Model file for the job. Use its own axes, mm. A direction names the side the tool comes from. Coordinates: 2 decimals unless noted, no trailing zeros. Write each loop counter-clockwise with the first axis right and the second up, starting at its lowest first coordinate (ties: lowest second). Pieces come first, ordered by that corner, then holes. Notation, with made-up numbers: (-26.75, 43) -> (24.25, 43) arc R14 cw to (24.25, 54) -> close; hole circle Ø10 at (13.5, -19.75). An arc over 180 degrees is marked (long way). Answer as a JSON object with one key per item and string values. Group by question number.
from build123d import *

# Parameters (mm, degrees)
EXTRUDE_2_DEPTH             = 20
HOLE_WIZARD_M41_D           = 4.5
HOLE_WIZARD_M41_DEPTH       = 6
HOLE_WIZARD_M41_CBORE_D     = 8
HOLE_WIZARD_M41_CBORE_DEPTH = 4
M4X0_71_D                   = 3.3
FILLET_1_R                  = 2
FILLET_2_R                  = 4
M4X0_72_D                   = 3.3
FILLET_3_R                  = 3


with BuildPart() as part:
    # Эскиз1 → Бобышка-Вытянуть2 (new body)
    with BuildSketch(Plane.XY):
        with BuildLine():
            Line((-6.608514495, 10.45), (6.608514495, 10.45))
            ThreePointArc((6.608514495, 10.45), (14.066074726, 13.916265053), (22.186198751, 12.614810542))
            Line((22.186198751, 12.614810542), (34.177275866, 33.383965344))
            Line((34.177275866, 33.383965344), (47.167656923, 25.883965344))
            Line((47.167656923, 25.883965344), (28.167656923, -7.025))
            ThreePointArc((28.167656923, -7.025), (23.025, -12.167656923), (16, -14.05))
            Line((16, -14.05), (-16, -14.05))
            ThreePointArc((-16, -14.05), (-23.025, -12.167656923), (-28.167656923, -7.025))
            Line((-28.167656923, -7.025), (-47.167656923, 25.883965344))
            Line((-47.167656923, 25.883965344), (-34.177275866, 33.383965344))
            Line((-34.177275866, 33.383965344), (-22.186198751, 12.614810542))
            ThreePointArc((-22.186198751, 12.614810542), (-14.066074726, 13.916265053), (-6.608514495, 10.45))
        make_face()
        with BuildLine():
            Line((-5.885653753, 4.45), (5.885653753, 4.45))
            ThreePointArc((5.885653753, 4.45), (27.047875471, -0.216673901), (5.71894947, -4.05))
            Line((5.71894947, -4.05), (-5.71894947, -4.05))
            ThreePointArc((-5.71894947, -4.05), (-27.047875471, -0.216673901), (-5.885653753, 4.45))
        make_face(mode=Mode.SUBTRACT)
    extrude(amount=EXTRUDE_2_DEPTH)

    # Цековка для винта с внутренним шестигранником M41
    with Locations(Plane(origin=(0, 10.45, 0), x_dir=(1, 0, 0), z_dir=(0, 1, 0))):
        with Locations((0, -10)):
            CounterBoreHole(HOLE_WIZARD_M41_D / 2, HOLE_WIZARD_M41_CBORE_D / 2, HOLE_WIZARD_M41_CBORE_DEPTH, depth=HOLE_WIZARD_M41_DEPTH)

    # Отверстие обработанное метчиком M4x0.71 (through all)
    with Locations(Plane(origin=(0, -4.05, 0), x_dir=(1, 0, 0), z_dir=(0, 1, 0))):
        with Locations((0, -10)):
            Hole(M4X0_71_D / 2)

    # Скругление1
    fillet_1_edges = [part.edges().sort_by_distance(p)[0] for p in [
        (-5.885653753, 4.45, 10),
        (-5.71894947, -4.05, 10),
        (5.71894947, -4.05, 10),
        (5.885653753, 4.45, 10),
    ]]
    fillet(fillet_1_edges, radius=FILLET_1_R)

    # Скругление2
    fillet_2_edges = [part.edges().sort_by_distance(p)[0] for p in [
        (-6.608514495, 10.45, 10),
        (6.608514495, 10.45, 10),
        (22.186198751, 12.614810542, 10),
        (-22.186198751, 12.614810542, 10),
    ]]
    fillet(fillet_2_edges, radius=FILLET_2_R)

    # Отверстие обработанное метчиком M4x0.72 (through all)
    with Locations(Plane(origin=(24.167656923, -13.95320323, 0), x_dir=(0, 0, -1), z_dir=(0.866025404, -0.5, 0))):
        with Locations((-10, 26), (-16, 38)):
            m4x0_72 = Hole(M4X0_72_D / 2)

    # Зеркальное отражение1: Отверстие обработанное метчиком M4x0.72 across plane
    add(m4x0_72.mirror(Plane(origin=(0, 0, 0), x_dir=(0, 0, 1), z_dir=(1, 0, 0))), mode=Mode.SUBTRACT)

    # Скругление3
    fillet_3_edges = [part.edges().sort_by_distance(p)[0] for p in [
        (34.177275866, 33.383965344, 10),
        (47.167656923, 25.883965344, 10),
        (-47.167656923, 25.883965344, 10),
        (-34.177275866, 33.383965344, 10),
    ]]
    fillet(fillet_3_edges, radius=FILLET_3_R)


solid = part.part
(1) Wall check: probe 1 along Z at (x, y) = (0, -8); probe 2 along Z at (x, y) = (0, 9.1); probe 3 along X at (y, z) = (-4.5, 5). Give the ranges that are in metal, low to high.
(2) Pull direction Z, two halves, no side cores. Call faces 1 (the face through (-3, 9, 20)), 2 (the face through (-36.829, 23.187, 17.574)), 3 (the face through (37.04, 8.34, 7.64)): released by +Z, released by -Z, zero draft, split by the parting line, or undercut.
(3) Cut at B-B on y = 0.5. List the corners of the cut face in (x, z).
(4) Cut at C-C on z = 16.25. Give the number of separate pieces and of enclosed holes in the cut face, plus the area to 3 significant figures.
(5) Pin check, flat tips, straight feed: pin 1 (8 mm diameter, centred on x = 9, z = 9.5, fed in from +Y); pin 2 (3 mm diameter, centred on y = 11.5, z = 17.5, fed in from +X); pin 3 (2 mm diameter, centred on x = 1, z = 5, fed in from +Y); pin 4 (3 mm diameter, centred on x = 0, z = 10, fed in from -Y). Stop position of each tip, or through.
(6) Cut at A-A on x = 0. List the corners of the cut face in (y, z), plus the area to 3 significant figures.
(7) 3-axis set-ups, long thin cutter, end or side, ignore diameter. For faces 4 (the face through (28.205, 23.04, 9.86)), 5 (the face through (-0.1, 4.45, 7.6)), 6 (the face through (0.29, 5.44, 7.77)): which of +Z, -Z, +X, -X, +Y, -Y reach the whole face in a straight line?
Results found:
{
 "1": {"probe 1": "z = 0 to 8.35, 11.65 to 20", "probe 2": "z = 0 to 6, 14 to 20", "probe 3": "x = -29.63 to -26.09, -5.7 to 5.7, 26.09 to 29.63"},
 "2": {"face 1": "released by +Z", "face 2": "undercut", "face 3": "zero draft"},
 "3": {"outline": "(-32.51, 0) -> (-27.04, 0) -> (-27.04, 20) -> (-32.51, 20) -> close; (27.04, 0) -> (32.51, 0) -> (32.51, 20) -> (27.04, 20) -> close"},
 "4": {"separate pieces": "3", "enclosed holes": "1", "area": "1,300 mm²"},
 "5": {"pin 1": "stops at y = 13.73", "pin 2": "stops at x = 39.73", "pin 3": "stops at y = 10.45", "pin 4": "passes through"},
 "6": {"outline": "(-14.05, 0) -> (-4.05, 0) -> (-4.05, 8.35) -> (-14.05, 8.35) -> close; (-14.05, 11.65) -> (-4.05, 11.65) -> (-4.05, 20) -> (-14.05, 20) -> close; (4.45, 0) -> (10.45, 0) -> (10.45, 6) -> (6.45, 6) -> (6.45, 7.75) -> (4.45, 7.75) -> close; (4.45, 12.25) -> (6.45, 12.25) -> (6.45, 14) -> (10.45, 14) -> (10.45, 20) -> (4.45, 20) -> close", "area": "246 mm²"},
 "7": {"face 4": "+Z, -Z, +Y", "face 5": "+Z, -Z", "face 6": "+Y"}
}
